Check sheet for the modelled part. Datum: model origin and axes. Units: mm. A direction names the side the tool comes from. Round coordinates to 2 decimals unless told otherwise and drop trailing zeros. Write each loop counter-clockwise with the first axis right and the second up, starting at its lowest first coordinate (ties: lowest second). Pieces come first, ordered by that corner, then holes. Notation, with made-up numbers: (6, 35) -> (61, 35) arc R25 cw to (61, 57) -> close; hole circle Ø4 at (49.5, 64). An arc over 180 degrees is marked (long way). Use one line per item in the form item = value. Start each with the question number.
```python
from build123d import *

# Parameters (mm, degrees)
F0_W     = 600
F0_H     = 400
F1_DEPTH = 250
F2_W     = 200
F2_H     = 200
F3_DEPTH = 250
F4_SIZE  = 199.99999


# Not quite as in the source:
# - a fillet or chamfer is up to 0.001 mm smaller than in the source, because OpenCascade refuses the exact size


with BuildPart() as f1:
    # F0 (on Top) → F1 (new body)
    with BuildSketch(Plane.XY):
        Rectangle(F0_W, F0_H)
    extrude(amount=F1_DEPTH)

    # F2 (on face) → F3 (join)
    with BuildSketch(Plane.XY.offset(250)):
        with Locations((0, 100)):
            Rectangle(F2_W, F2_H)
    extrude(amount=F3_DEPTH)

    # F4 (size 200 in the source; OpenCascade refuses exactly that, so slightly less here)
    f4_edges = [f1.edges().sort_by_distance(p)[0] for p in [
        (0, -200, 250),
    ]]
    chamfer(f4_edges, length=F4_SIZE)


solid = f1.part
```
1. Scan lines: probe 1 along X at (y, z) = (91, 276.5); probe 2 along Z at (x, y) = (139, 44.5); probe 3 along Y at (x, z) = (-84.5, 432). Record each from-to range of solid material in increasing order.
2. Sectioned sample at C-C (z = 443.5). Enter the section's corners in (x, y), and give its area (3 significant figures).
3. Sectioned sample at D-D (x = -229.5). Enter the section's corners in (y, z), and give its area (3 significant figures).
4. Depth check by flat-ended pin: pin 1 (1.5 mm diameter, centred on y = 122.5, z = 397, fed in from +X); pin 2 (8 mm diameter, centred on x = -208, y = -137.5, fed in from +Z); pin 3 (1.5 mm diameter, centred on x = 163, z = 242, fed in from -Y). Enter the tip coordinate at first touch or a pass-through.
5. Sectioned sample at B-B (y = 150.5). Enter the section's corners in (x, z).
6. Tool access check on faces 1 (the face through (-1, 0, 373)), 2 (the face through (-100, 99, 373)), 3 (the face through (-138, 101, 250)), 4 (the face through (100, 99, 373)). Record the directions out of +Z, -Z, +X, -X, +Y, -Y that give a thin tool (end or side, any length) a straight path to the whole face; none if there is none.
Returned:
q1.probe_1 = -100 to 100
q1.probe_2 = 0 to 250
q1.probe_3 = 0 to 200
q2.outline = (-100, 0) -> (100, 0) -> (100, 200) -> (-100, 200) -> close
q2.area = 40,000 mm^2
q3.outline = (-200, 0) -> (200, 0) -> (200, 250) -> (0, 250) -> (-200, 50) -> close
q3.area = 80,000 mm^2
q4.pin_1 = 100
q4.pin_2 = 116.5
q4.pin_3 = -8.75
q5.outline = (-300, 0) -> (300, 0) -> (300, 250) -> (100, 250) -> (100, 500) -> (-100, 500) -> (-100, 250) -> (-300, 250) -> close
q6.face_1 = +Z, +X, -X, -Y
q6.face_2 = +Z, -X, +Y, -Y
q6.face_3 = +Z, -X, +Y, -Y
q6.face_4 = +Z, +X, +Y, -Y
